Here's how the part is built. I have some questions about the finished solid (model axes, mm). Face numbers are marked on the shaded views. Coordinates: 2 decimals unless noted, no trailing zeros. Write each loop counter-clockwise with the first axis right and the second up, starting at its lowest first coordinate (ties: lowest second). Pieces come first, ordered by that corner, then holes.
Item 1: If I drill on line 1 (Y direction, x = 7, z = 4.5); line 2 (Z direction, x = 22, y = 20); line 3 (X direction, y = -21, z = 7), over which ranges is the centre line in solid material (lowest first)?
Item 2: I'm going to push flat-ended pins straight in: pin 1 Ø3 at (x, y) = (-3, -19.5) entering from +Z; pin 2 Ø2 at (y, z) = (-4, 4.5) entering from -X. Where does each tip first touch, or does it pass through?
Item 3: If we section it at C-C (y = -5): Please give me the cut outline in (x, z), then the cut area to 3 significant figures.
Item 4: We'd pull the mould along Y, two halves only. Please class the marked faces 1, 2, 3 and 4: +Y half, -Y half, draft (parallel to the pull), parting line (faces both ways), or undercut.
Item 5: If we section it at B-B (z = 3.25): Please give me the cut outline in (x, y), then the cut area to 3 significant figures.
Item 6: If we section it at A-A (x = 6.5): Please give me the cut outline in (y, z).
from build123d import *

# Parameters (mm, degrees)
F0_W           = 90
F0_H           = 72
F1_DEPTH       = 8
F2_W           = 87.5752791762
F2_H           = 69.5543810725
F3_DEPTH       = 7
F5_D           = 7
F5_CBORE_D     = 7
F5_CBORE_DEPTH = 1
F7_DEPTH       = 2


with BuildPart() as f1:
    # F0 (on Top) → F1 (new body)
    with BuildSketch(Plane.XY):
        with Locations((-1.6035065055, 0.9231414078)):
            Rectangle(F0_W, F0_H)
    extrude(amount=F1_DEPTH)

    # F2 (on face) → F3 (cut)
    with BuildSketch(Plane.XY.offset(8)):
        with Locations((-1.6968734562, 1.0423921049)):
            Rectangle(F2_W, F2_H)
    extrude(amount=-F3_DEPTH, mode=Mode.SUBTRACT)

    # F5 (through all)
    with Locations(Plane(origin=(-46.6035065055, 0, 0), x_dir=(0, -1, 0), z_dir=(-1, 0, 0))):
        with Locations((0, 5.0745382905)):
            CounterBoreHole(F5_D / 2, F5_CBORE_D / 2, F5_CBORE_DEPTH)

    # F6 (on face) → F7 (cut)
    with BuildSketch(Plane(origin=(-46.6035065055, 0, 0), x_dir=(0, -1, 0), z_dir=(-1, 0, 0))):
        with BuildLine():
            Line((-36.9231414078, 8), (-36.9231414078, 0))
            Line((-36.9231414078, 0), (35.0768585922, 0))
            Line((35.0768585922, 0), (35.0768585922, 8))
            Line((35.0768585922, 8), (1.921372891, 8))
            ThreePointArc((1.921372891, 8), (0, 1.5745382905), (-1.921372891, 8))
            Line((-1.921372891, 8), (-36.9231414078, 8))
        make_face()
    extrude(amount=-F7_DEPTH, mode=Mode.SUBTRACT)


solid = f1.part
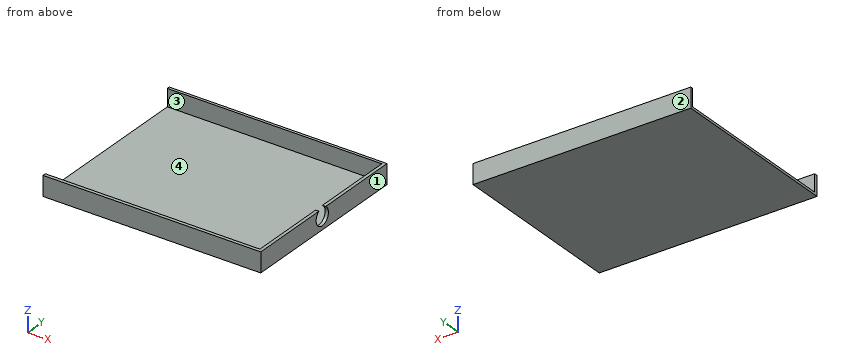
Answer list:
1. line 1: y = -35.08 to -33.73, 35.82 to 36.92
1. line 2: z = 0 to 1
1. line 3: x = 42.09 to 43.4
2. pin 1: stops at z = 1
2. pin 2: stops at x = 42.09
3. outline: (-44.6, 0) - (43.4, 0) - (43.4, 8) - (42.09, 8) - (42.09, 1) - (-44.6, 1) - close
3. area: 97.1 mm2
4. face 1: draft
4. face 2: +Y half
4. face 3: undercut
4. face 4: undercut
5. outline: (-44.6, -35.08) - (43.4, -35.08) - (43.4, -2.99) - (42.09, -2.99) - (42.09, -33.73) - (-44.6, -33.73) - close; (-44.6, 35.82) - (42.09, 35.82) - (42.09, 2.99) - (43.4, 2.99) - (43.4, 36.92) - (-44.6, 36.92) - close
5. area: 298 mm2
6. outline: (-35.08, 0) - (36.92, 0) - (36.92, 8) - (35.82, 8) - (35.82, 1) - (-33.73, 1) - (-33.73, 8) - (-35.08, 8) - close
